The figure shows three views and two pictorial views of one solid part (mm, origin at its lowest corner). Answer the questions. A direction names the side the tool comes from. Round coordinates to 2 decimals unless told otherwise and drop trailing zeros. Order: outer loops, then holes, each group sorted by start corner. A loop starts at its lowest first (then second) coordinate and runs counter-clockwise, first axis right, second up. Notation, with made-up numbers: M 56.25,-10 L 110.25,-10 A13 cw 110.25,2 Z; hole C 86.5,20.25 d10. An arc over 180 degrees is marked long. Return JSON: item names as keys, results as strings.
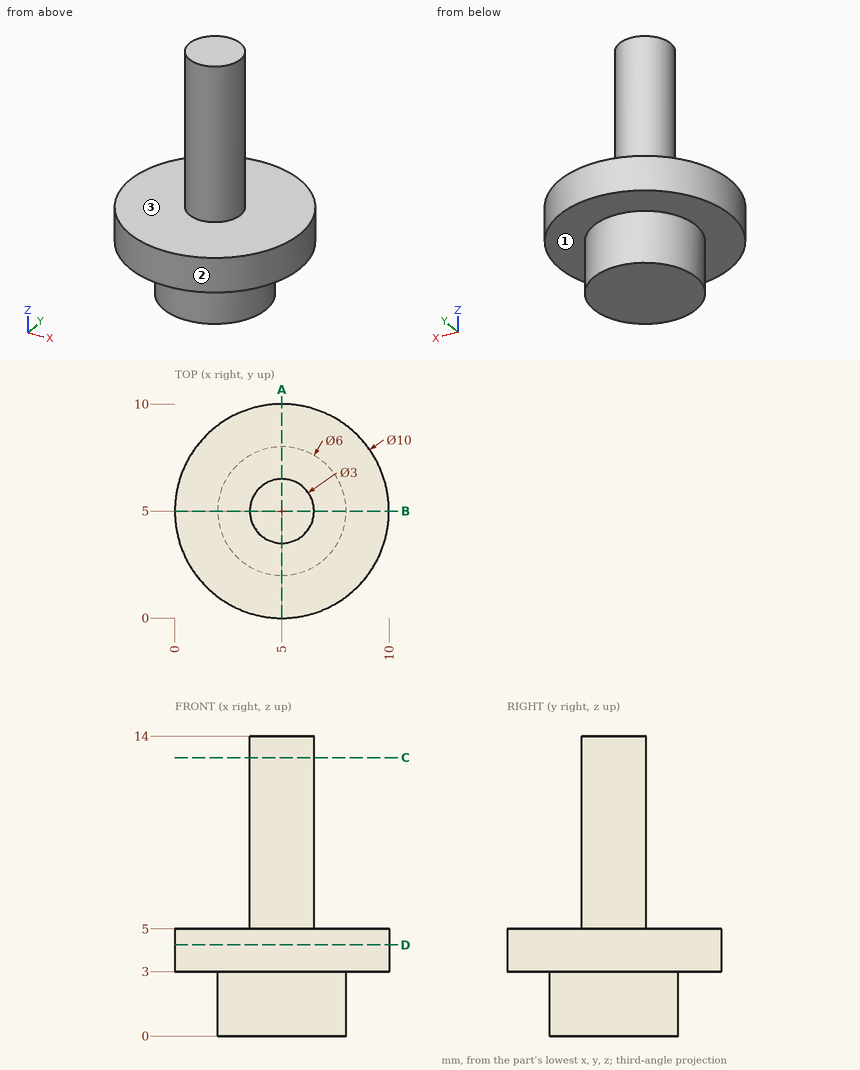
Item 1: Which of the six approach directions +Z, -Z, +X, -X, +Y, -Y give full straight-line access (tool end or side, diameter ignored) to the marked faces 1, 2 and 3?
Output:
{"face 1": "-Z", "face 2": "+Z, -Z", "face 3": "+Z"}
Item 2: Consider line 1 along Z through (x, y) = (3.5, 7); line 2 along X through (y, z) = (5, 6.5); line 3 along Z through (x, y) = (8.5, 2.5). Determine where each line is inside the solid, lowest interval first. Write a range as [from, to].
Output:
{"line 1": "z = [0, 5]", "line 2": "x = [3.5, 6.5]", "line 3": "z = [3, 5]"}
Item 3: Find section C-C (z = 13). Determine the outline of the cut face in (x, y).
Output:
{"outline": "C 5,5 d3"}
Item 4: Find section A-A (x = 5). Determine the outline of the cut face in (y, z).
Output:
{"outline": "M 0,3 L 2,3 L 2,0 L 8,0 L 8,3 L 10,3 L 10,5 L 6.5,5 L 6.5,14 L 3.5,14 L 3.5,5 L 0,5 Z"}
Item 5: Each of these flat-tipped pins is pushed along its axis until it touches: pin 1 (1 mm diameter, centred on x = 2.5, z = 8, fed in from +Y); pin 2 (3 mm diameter, centred on x = 4, z = 12, fed in from -Y); pin 3 (1.5 mm diameter, centred on y = 6, z = 12, fed in from -X). Where does it stop, or does it pass through?
Output:
{"pin 1": "passes through", "pin 2": "stops at y = 3.5", "pin 3": "stops at x = 3.52"}
Item 6: Find section D-D (z = 4.25). Determine the outline of the cut face in (x, y).
Output:
{"outline": "C 5,5 d10"}
